Check sheet for the modelled part. Datum: model origin and axes. Units: mm. A direction names the side the tool comes from. Round coordinates to 2 decimals unless told otherwise and drop trailing zeros. Loops run counter-clockwise (first coordinate to the right, second up) from the corner with the lowest first, then second, coordinate; pieces in that order, holes last. Notation, with made-up numbers: (-6, -8.5) -> (27, -8.5) arc R8 cw to (27, -3.5) -> close; hole circle Ø4 at (0, 28). An arc over 180 degrees is marked (long way). Return JSON: item names as keys, results as strings.
from build123d import *

# Parameters (mm, degrees)
SKETCH1_R             = 29
SKETCH1_R_2           = 14.5
SKETCH1_R_3           = 1
BOSS_EXTRUDE1_DEPTH   = 3
SKETCH2_R             = 19
SKETCH2_R_2           = 16
BOSS_EXTRUDE2_DEPTH   = 9
F_6_0MM_DOWEL_HOLE1_D = 6
CHAMFER1_SIZE         = 0.5


with BuildPart() as part:
    # Sketch1 → Boss-Extrude1 (new body)
    with BuildSketch(Plane(origin=(0, 0, 0), x_dir=(1, 0, 0), z_dir=(0, 1, 0))):
        with Locations(Location((0, 0, 0), (0, 0, 270))):
            Circle(SKETCH1_R)
        with Locations(Location((0, 0, 0), (0, 0, 270))):
            Circle(SKETCH1_R_2, mode=Mode.SUBTRACT)
        with Locations(Location((0, 24, 0), (0, 0, 270))):
            Circle(SKETCH1_R_3, mode=Mode.SUBTRACT)
        with Locations(Location((24, 0, 0), (0, 0, 270))):
            Circle(SKETCH1_R_3, mode=Mode.SUBTRACT)
        with Locations(Location((0, -24, 0), (0, 0, 270))):
            Circle(SKETCH1_R_3, mode=Mode.SUBTRACT)
        with Locations(Location((-24, 0, 0), (0, 0, 270))):
            Circle(SKETCH1_R_3, mode=Mode.SUBTRACT)
    extrude(amount=BOSS_EXTRUDE1_DEPTH)

    # Sketch2 → Boss-Extrude2 (add)
    with BuildSketch(Plane(origin=(0, 3, 0), x_dir=(1, 0, 0), z_dir=(0, 1, 0))):
        with Locations(Location((0, 0, 0), (0, 0, 270))):
            Circle(SKETCH2_R)
        with Locations(Location((0, 0, 0), (0, 0, 270))):
            Circle(SKETCH2_R_2, mode=Mode.SUBTRACT)
    extrude(amount=BOSS_EXTRUDE2_DEPTH)

    # Ø6.0mm Dowel Hole1 (through all)
    with Locations(Plane(origin=(0, 3, 0), x_dir=(1, 0, 0), z_dir=(0, 1, 0))):
        with Locations((0, 24), (24, 0), (0, -24), (-24, 0)):
            Hole(F_6_0MM_DOWEL_HOLE1_D / 2)

    # Chamfer1
    chamfer1_edges = [part.edges().sort_by_distance(p)[0] for p in [
        (0, 12, -16),
    ]]
    chamfer(chamfer1_edges, length=CHAMFER1_SIZE)


solid = part.part
Q1. Go/stop test with flat-tipped pins: pin 1 (6 mm diameter, centred on y = 9.5, z = 19.5, fed in from -X); pin 2 (5 mm diameter, centred on y = 4, z = -19.5, fed in from -X); pin 3 (5 mm diameter, centred on x = -3.5, y = 7, fed in from +Z). Record where each tip stops, or that it passes through.
Results list:
{"pin 1": "x = -9.42", "pin 2": "x = -23.34", "pin 3": "z = 18.97"}
Q2. Tool access check on faces 1 (the flat face through (-19, 3, 6)), 2 (the flat face through (16, 12, -6)). Record the directions out of +Z, -Z, +X, -X, +Y, -Y that give a thin tool (end or side, any length) a straight path to the whole face; none if there is none.
Results list:
{"face 1": "+Y", "face 2": "+Z, -Z, +X, -X, +Y"}
Q3. Draft check along Z on faces 3 (the cylindrical face through (-11.107, 1.479, 26.789)), 4 (the flat face through (7, 0, -13)), 5 (the cylindrical face through (-5.554, 1.479, 13.394)). Enter one of: released by +Z, released by -Z, zero draft, split by the parting line, or undercut.
Results list:
{"face 3": "split by the parting line", "face 4": "zero draft", "face 5": "undercut"}
Q4. Section check A-A (x = 0). Record the boundary of the cut face in (y, z).
Results list:
{"outline": "(0, -29) -> (3, -29) -> (3, -27) -> (0, -27) -> close; (0, -21) -> (3, -21) -> (3, -19) -> (12, -19) -> (12, -16.5) -> (11.5, -16) -> (3, -16) -> (3, -14.5) -> (0, -14.5) -> close; (0, 14.5) -> (3, 14.5) -> (3, 16) -> (11.5, 16) -> (12, 16.5) -> (12, 19) -> (3, 19) -> (3, 21) -> (0, 21) -> close; (0, 27) -> (3, 27) -> (3, 29) -> (0, 29) -> close"}
Q5. Material ranges on line 1 (X direction, y = 9.75, z = 0); line 2 (Y direction, x = 12, z = 18); line 3 (X direction, y = 4.5, z = 11), recorded low to high.
Results list:
{"line 1": "-19 to -16, 16 to 19", "line 2": "0 to 3", "line 3": "-15.49 to -11.62, 11.62 to 15.49"}
Q6. Section check D-D (x = 24). Record the boundary of the cut face in (y, z), then the cut area to 3 significant figures.
Results list:
{"outline": "(0, -16.28) -> (3, -16.28) -> (3, -3) -> (0, -3) -> close; (0, 3) -> (3, 3) -> (3, 16.28) -> (0, 16.28) -> close", "area": "79.7 mm^2"}
Q7. Section check C-C (y = 1.25). Record the boundary of the cut face in (x, z).
Results list:
{"outline": "circle Ø58 at (0, 0); hole circle Ø6 at (-24, 0); hole circle Ø29 at (0, 0); hole circle Ø6 at (0, -24); hole circle Ø6 at (0, 24); hole circle Ø6 at (24, 0)"}
Q8. Section check B-B (z = 0). Record the boundary of the cut face in (x, y).
Results list:
{"outline": "(-29, 0) -> (-27, 0) -> (-27, 3) -> (-29, 3) -> close; (-21, 0) -> (-14.5, 0) -> (-14.5, 3) -> (-16, 3) -> (-16, 11.5) -> (-16.5, 12) -> (-19, 12) -> (-19, 3) -> (-21, 3) -> close; (14.5, 0) -> (21, 0) -> (21, 3) -> (19, 3) -> (19, 12) -> (16.5, 12) -> (16, 11.5) -> (16, 3) -> (14.5, 3) -> close; (27, 0) -> (29, 0) -> (29, 3) -> (27, 3) -> close"}
